Solid Edge part; units mm, degrees
sketch "Sketch1" plane through (0, 0, 0) normal (0, -1, 0) x (1, 0, 0)
  line L0 (-94.9915, 16.9957) -> (225.0085, 16.9957)
  line L1 (225.0085, 16.9957) -> (225.0085, 50.4601)
  line L2 (225.0085, 50.4601) -> (-94.9915, 50.4601)
  line L3 (-94.9915, 50.4601) -> (-94.9915, 16.9957)
  dimension "D1" = 225.0085
  dimension "D2" = 94.9915
extrude "Protrusion1" add sketch "Sketch1" along normal blind 80
sketch "Sketch2" plane through (55.0085, -15, 50.4601) normal (0, 0, 1) x (1, 0, 0)
  line L0 (-140, -12.3571) -> (160, -12.3571)
  line L1 (160, -12.3571) -> (160, 5)
  line L2 (160, 5) -> (-140, 5)
  line L3 (-140, 5) -> (-140, -12.3571)
  dimension "D1" = 160
  dimension "D2" = 160
extrude "Cutout1" cut sketch "Sketch2" against normal through all
sketch "Sketch3" plane through (65.0085, -80, 33.7279) normal (0, -1, 0) x (1, 0, 0)
  circle A0 centre (70, -5) radius 5
  circle A1 centre (-80, -5) radius 5
extrude "Cutout2" cut sketch "Sketch3" against normal through all
Input: part model. Units: mm. Frame: model coordinates. A direction names the side the tool comes from. Give positions to 0.01 mm unless a question says otherwise; leave off trailing zeros. Write each loop counter-clockwise with the first axis right and the second up, starting at its lowest first coordinate (ties: lowest second). Pieces come first, ordered by that corner, then holes. Notation, with made-up numbers: (67.5, -8) - (101.5, -8) arc R14 ccw to (101.5, 11) - close; hole circle Ø4 at (-25, 26). An arc over 180 degrees is marked (long way). Write item = value, one per line. Start each with the question number.
1. Section query A-A, the plane y = -23. Output: boundary loops of the cut face in (x, z).
2. Access query for faces 1 (the flat face through (215.008, -19, 34)), 2 (the flat face through (67, -80, 34)). Directions: +Z, -Z, +X, -X, +Y, -Y. A direction counts if a zero-diameter tool reaches every point of the face in a straight line with its end or side. Return the directions, or none.
3. Section query C-C, the plane x = 92. Output: boundary loops of the cut face in (y, z).
4. Mould query, pull axis Y, two halves, no side actions, for faces 3 (the flat face through (67, 0, 34)), 4 (the flat face through (-84.992, -19, 34)), 5 (the flat face through (63, -48, 16.996)). Classes: released by +Y, released by -Y, zero draft, split by the parting line, or undercut.
5. First-contact query: pin 1 Ø10 at (x, z) = (117.5, 36.5) entering from +Y. Flat tip, straight axial feed; report the tip coordinate or a pass-through.
6. Section query B-B, the plane z = 45.5. Output: boundary loops of the cut face in (x, y), then the cut area to 3 significant figures.
7. Ray query, L1, parallel to X at y = -13.5, z = 44; L2, parallel to Y at x = 17.5, z = 20.5; L3, parallel to X at y = -29, z = 28.5. Return the intervals inside material, ascending.
Check sheet entries:
q1.outline = (-94.99, 17) - (-84.99, 17) - (-84.99, 50.46) - (-94.99, 50.46) - close; (215.01, 17) - (225.01, 17) - (225.01, 50.46) - (215.01, 50.46) - close
q2.face_1 = +Z, -Z
q2.face_2 = +Z, -Z, +X, -X, -Y
q3.outline = (-80, 17) - (-27.36, 17) - (-27.36, 50.46) - (-80, 50.46) - close; (-10, 17) - (0, 17) - (0, 50.46) - (-10, 50.46) - close
q4.face_3 = released by +Y
q4.face_4 = undercut
q4.face_5 = zero draft
q5.pin_1 = 0
q6.outline = (-94.99, -80) - (225.01, -80) - (225.01, 0) - (-94.99, 0) - close; hole (-84.99, -27.36) - (215.01, -27.36) - (215.01, -10) - (-84.99, -10) - close
q6.area = 20,400 mm2
q7.L1 = -94.99 to -84.99, 215.01 to 225.01
q7.L2 = -80 to -27.36, -10 to 0
q7.L3 = -94.99 to -19.99, -10 to 130.01, 140 to 225.01
